Work out the finished part from the listing and answer in its coordinate system (mm). Face numbers are marked on the shaded views. A direction names the side the tool comes from. Round coordinates to 2 decimals unless told otherwise and drop trailing zeros. Order: outer loops, then holes, each group sorted by start corner. A loop starts at its lowest first (then second) coordinate and runs counter-clockwise, first axis right, second up. Notation, with made-up numbers: (2.25, -14) -> (51.25, -14) arc R32 cw to (51.25, 25) -> close; hole circle Ø6 at (68.25, 44). An arc over 180 degrees is marked (long way). Use a Markdown table: item, result. Add a question column.
Item 1: A tool of negligible diameter and unlimited length cuts with its end or side. For the marked faces 5, 6 and 7, from which of +Z, -Z, +X, -X, +Y, -Y can it reach the whole face along a straight path? Write none if from no direction.
Item 2: A cutting plane is placed at D-D, the plane z = -80.5. Determine the outline of the cut face in (x, y), plus the area to 3 significant figures.
Item 3: Flat-ended cylindrical pins translate along their axes: P1, Ø1, axis at x = -85, y = -100.5, coming from the +Z side; P2, Ø10.5, axis at y = -95, z = -45.5, coming from the -X side; P3, Ø17.5, axis at y = -100, z = -19, coming from the +X side. Find the tip coordinate at first contact, or state that the pin passes through.
Item 4: For a pull along Z with two mould halves and no side action, classify the marked faces 1, 2, 3 and 4 as +Z half, -Z half, draft (parallel to the pull), parting line (faces both ways), or undercut.
Item 5: A cutting plane is placed at A-A, the plane z = -44. Determine the outline of the cut face in (x, y).
Item 6: Find the intervals of material crossed by L1, parallel to Z at x = -92, y = -101.5; L2, parallel to Z at x = -84.5, y = -106; L3, parallel to Z at x = -95.5, y = -97, in increasing order. Write a range as [from, to].
Item 7: A cutting plane is placed at B-B, the plane x = -64. Determine the outline of the cut face in (y, z).
Item 8: A cutting plane is placed at C-C, the plane y = -85. Determine the outline of the cut face in (x, z), plus the area to 3 significant figures.
from build123d import *

# Parameters (mm, degrees)
EXTRUDE_1_DEPTH     = 10
EXTRUDE_3_DEPTH     = 40
FILLET_2_R          = 3
FILLET_3_R          = 3
SKETCH_10_W         = 43.3
SKETCH_10_H         = 35
CUT_EXTRUDE_1_DEPTH = 12.8
EXTRUDE_4_DEPTH     = 35


with BuildPart() as part:
    # 草图3 → 凸台-拉伸1 (new body)
    with BuildSketch(Plane.XY):
        Polygon((-100, -79.175359259), (-100, -119.175359259), (-60, -119.175359259), (-60, -114.175359259), (-95, -79.175359259), align=None)
    extrude(amount=-EXTRUDE_1_DEPTH)

    # 草图5 → 切除-放样1 section 0
    with BuildSketch(Plane.XY.offset(-6)):
        with BuildLine():
            Line((-96.08, -104.799041882), (-96.08, -98.821989002))
            Line((-96.08, -98.821989002), (-81.709132385, -81.695455893))
            Line((-81.709132385, -81.695455893), (-66.265676412, -94.654054104))
            Line((-66.265676412, -94.654054104), (-83.579668035, -115.288065824))
            Line((-83.579668035, -115.288065824), (-96.08, -104.799041882))
        make_face()
    # 草图8 → 切除-放样1 section 1
    with BuildSketch(Plane.XY):
        with BuildLine():
            Line((-94.58, -104.099580395), (-94.58, -99.367944353))
            Line((-94.58, -99.367944353), (-80.56006572, -82.659637307))
            Line((-80.56006572, -82.659637307), (-67.414743077, -93.68987269))
            Line((-67.414743077, -93.68987269), (-83.764553285, -113.174817744))
            Line((-83.764553285, -113.174817744), (-94.58, -104.099580395))
        make_face()
    loft(mode=Mode.SUBTRACT)

    # 草图9 → 凸台-拉伸3 (add)
    with BuildSketch(Plane(origin=(0, 0, -10), x_dir=(-1, 0, 0), z_dir=(0, 0, -1))):
        Polygon((95, -79.175359259), (95, -114.175359259), (60, -114.175359259), (60, -119.175359259), (100, -119.175359259), (100, -79.175359259), align=None)
    extrude(amount=EXTRUDE_3_DEPTH)

    # 镜向2: part across plane


with BuildPart() as part_1:
    add(part.part)
    add(part.part.mirror(Plane(origin=(0, 0, -50), x_dir=(1, 0, 0), z_dir=(0, 0, -1))))

    # 圆角2
    fillet_2_edges = [part_1.edges().sort_by_distance(p)[0] for p in [
        (-60, -116.675359259, -100),
        (-60, -116.675359259, 0),
        (-100, -99.175359259, -100),
        (-100, -99.175359259, 0),
        (-100, -79.175359259, -50),
        (-97.5, -79.175359259, 0),
    ]]
    fillet(fillet_2_edges, radius=FILLET_2_R)

    # 圆角3
    fillet_3_edges = [part_1.edges().sort_by_distance(p)[0] for p in [
        (-80, -119.175359259, -100),
        (-80, -119.175359259, 0),
        (-100, -119.175359259, -50),
        (-60, -119.175359259, -50),
        (-99.121320344, -119.175359259, -0.878679656),
        (-99.121320344, -119.175359259, -99.121320344),
        (-60.878679656, -119.175359259, -0.878679656),
        (-60.878679656, -119.175359259, -99.121320344),
    ]]
    fillet(fillet_3_edges, radius=FILLET_3_R)

    # 草图10 → 切除-拉伸1 (cut)
    with BuildSketch(Plane.ZY.offset(100)):
        with Locations((-51.5, -96.675359259)):
            Rectangle(SKETCH_10_W, SKETCH_10_H)
    extrude(amount=-CUT_EXTRUDE_1_DEPTH, mode=Mode.SUBTRACT)

    # 草图11 → 凸台-拉伸4 (add)
    with BuildSketch(Plane(origin=(0, -114.175359259, 0), x_dir=(1, 0, 0), z_dir=(0, 1, 0))):
        Polygon((-95, 25.85), (-83, 25.85), (-83, 77.15), (-95, 77.15), (-95, 73.15), (-87, 73.15), (-87, 29.85), (-95, 29.85), align=None)
    extrude(amount=EXTRUDE_4_DEPTH)


solid = part_1.part
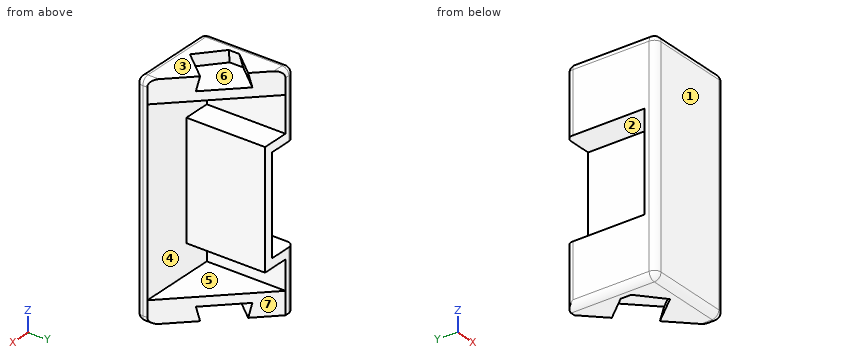
Reported:
| question | item | result |
|---|---|---|
| 1 | face 5 | +X, +Y |
| 1 | face 6 | none |
| 1 | face 7 | -Z, +X, +Y |
| 2 | outline | (-100, -116.18) arc R3 ccw to (-97, -119.18) -> (-63, -119.18) arc R3 ccw to (-60, -116.18) -> (-60, -114.18) -> (-95, -114.18) -> (-95, -79.18) -> (-97, -79.18) arc R3 ccw to (-100, -82.18) -> close |
| 2 | area | 369 mm² |
| 3 | P1 | z = -6 |
| 3 | P2 | x = -87 |
| 3 | P3 | x = -83 |
| 4 | face 1 | draft |
| 4 | face 2 | undercut |
| 4 | face 3 | +Z half |
| 4 | face 4 | undercut |
| 5 | outline | (-100, -116.18) arc R3 ccw to (-97, -119.18) -> (-63, -119.18) arc R3 ccw to (-60, -116.18) -> (-60, -114.18) -> (-83, -114.18) -> (-83, -79.18) -> (-87, -79.18) -> (-87, -114.18) -> (-100, -114.18) -> close |
| 6 | L1 | [-94, -90], [-77.15, -73.15], [-29.85, -25.85], [-10, -6] |
| 6 | L2 | [-94, -90], [-77.15, -25.85], [-10, -6] |
| 6 | L3 | [-100, -73.15], [-29.85, 0] |
| 7 | outline | (-119.18, -97) arc R3 ccw to (-116.18, -100) -> (-110.18, -100) -> (-110.18, -90) -> (-114.18, -90) -> (-114.18, -10) -> (-110.18, -10) -> (-110.18, 0) -> (-116.18, 0) arc R3 ccw to (-119.18, -3) -> close |
| 8 | outline | (-100, -97) arc R3 ccw to (-97, -100) -> (-89.18, -100) -> (-89.18, -90) -> (-95, -90) -> (-95, -77.15) -> (-83, -77.15) -> (-83, -25.85) -> (-95, -25.85) -> (-95, -10) -> (-89.18, -10) -> (-89.18, 0) -> (-97, 0) arc R3 ccw to (-100, -3) -> (-100, -29.85) -> (-87, -29.85) -> (-87, -73.15) -> (-100, -73.15) -> close |
| 8 | area | 665 mm² |
